```python
from build123d import *

# Parameters (mm, degrees)
F0_W     = 525
F0_H     = 670
F1_DEPTH = 21
F2_R     = 206
F3_DEPTH = 25


with BuildPart() as f1:
    # F0 (on Front) → F1 (new body)
    with BuildSketch(Plane.XZ):
        Rectangle(F0_W, F0_H)
    extrude(amount=F1_DEPTH)

    # F2 (on face) → F3 (cut)
    with BuildSketch(Plane.XZ.offset(21)):
        with Locations((0, 35)):
            Circle(F2_R)
    extrude(amount=-F3_DEPTH, mode=Mode.SUBTRACT)


solid = f1.part
```
The listing builds one solid part. Answer for the finished solid, in the listing's coordinates (mm). Coordinates: 2 decimals unless noted, no trailing zeros. Loops run counter-clockwise (first coordinate to the right, second up) from the corner with the lowest first, then second, coordinate; pieces in that order, holes last. Notation, with made-up numbers: (51.25, -5.5) - (62.25, -5.5) arc R14 cw to (62.25, 12.5) - close; hole circle Ø1 at (-10.5, -4.5). An arc over 180 degrees is marked (long way). Use a Markdown table: item, result. Add a question column.
1) The mould has two halves that part along X. Classify faces 1 (the flat face through (-120, 0, -144)), 2 (the cylindrical face through (-44.66, -10.65, -166.1)), 3 (the flat face through (-262.5, -10, -5)): released by +X, released by -X, zero draft, split by the parting line, or undercut.
2) The part is cut by section B-B, the plane x = 0. Give the vertices of the cut face in (y, z).
3) The part is cut by section C-C, the plane y = -4.75. Give the vertices of the cut face in (x, z).
4) The part is cut by section A-A, the plane z = 35. Give the vertices of the cut face in (x, y).
5) Find the intervals of material crossed by line 1 (X direction, y = -13.25, z = 34); line 2 (Z direction, x = 0, y = -11.5); line 3 (Z direction, x = 59, y = -13.25), in increasing order.
6) Given pin 1 (3 mm diameter, centred on x = -167.5, z = 171.5, fed in from +Y), flat-ended and moving along its own axis, determine where the tip first touches the part or whether it passes through.
Here are the results:
| question | item | result |
|---|---|---|
| 1 | face 1 | zero draft |
| 1 | face 2 | undercut |
| 1 | face 3 | released by -X |
| 2 | outline | (-21, -335) - (0, -335) - (0, -171) - (-21, -171) - close; (-21, 241) - (0, 241) - (0, 335) - (-21, 335) - close |
| 3 | outline | (-262.5, -335) - (262.5, -335) - (262.5, 335) - (-262.5, 335) - close; hole circle Ø412 at (0, 35) |
| 4 | outline | (-262.5, -21) - (-206, -21) - (-206, 0) - (-262.5, 0) - close; (206, -21) - (262.5, -21) - (262.5, 0) - (206, 0) - close |
| 5 | line 1 | x = -262.5 to -206, 206 to 262.5 |
| 5 | line 2 | z = -335 to -171, 241 to 335 |
| 5 | line 3 | z = -335 to -162.37, 232.37 to 335 |
| 6 | pin 1 | stops at y = 0 |
